```python
from build123d import *

# Parameters (mm, degrees)
SKETCH1_W            = 37
SKETCH1_H            = 57
SKETCH1_W_2          = 22
SKETCH1_H_2          = 42
BOSS_EXTRUDE1_DEPTH  = 5
M4_CLEARANCE_HOLE1_D = 4.5
SKETCH4_W            = 5
SKETCH4_H            = 57
BOSS_EXTRUDE2_DEPTH  = 30


with BuildPart() as part:
    # Sketch1 → Boss-Extrude1 (new body)
    with BuildSketch(Plane(origin=(0, 0, 0), x_dir=(1, 0, 0), z_dir=(0, 1, 0))):
        Rectangle(SKETCH1_W, SKETCH1_H)
        Rectangle(SKETCH1_W_2, SKETCH1_H_2, mode=Mode.SUBTRACT)
    extrude(amount=BOSS_EXTRUDE1_DEPTH)

    # M4 Clearance Hole1 (through all)
    with Locations(Plane(origin=(0, 5, 0), x_dir=(1, 0, 0), z_dir=(0, 1, 0))):
        with Locations((-6.3, 24.2), (6.3, 24.2), (-6.3, -24.2), (6.3, -24.2)):
            Hole(M4_CLEARANCE_HOLE1_D / 2)

    # Sketch4 → Boss-Extrude2 (add)
    with BuildSketch(Plane(origin=(0, 0, 0), x_dir=(1, 0, 0), z_dir=(0, 1, 0))):
        with Locations((-21, 0)):
            Rectangle(SKETCH4_W, SKETCH4_H)
        with Locations((21, 0)):
            Rectangle(SKETCH4_W, SKETCH4_H)
    extrude(amount=BOSS_EXTRUDE2_DEPTH)


solid = part.part
```
Verification items for the finished model (mm, model axes). A direction names the side the tool comes from. Coordinates: 2 decimals unless noted, no trailing zeros. Order: outer loops, then holes, each group sorted by start corner. A loop starts at its lowest first (then second) coordinate and runs counter-clockwise, first axis right, second up. Notation, with made-up numbers: (56.25, -13.75) - (66.25, -13.75) arc R19 cw to (66.25, -2.75) - close; hole circle Ø9 at (-31, -7). An arc over 180 degrees is marked (long way). Return JSON: item names as keys, results as strings.
(1) Section check B-B, the plane y = 23.5. Record the cut outline in (x, z).
Filled sheet:
{"outline": "(-23.5, -28.5) - (-18.5, -28.5) - (-18.5, 28.5) - (-23.5, 28.5) - close; (18.5, -28.5) - (23.5, -28.5) - (23.5, 28.5) - (18.5, 28.5) - close"}
(2) Mould release check, pull along Z, two halves, no side actions. Record for faces 4 (the flat face through (11, 2, 0)), 5 (the flat face through (-11, 2, 0)), 6 (the flat face through (-0.3, 4.8, 28.5)), 7 (the flat face through (-18.5, 17, 0)): pulls with the +Z half, pulls with the -Z half, needs draft (parallel to the pull), parting line crosses it, or undercut.
Filled sheet:
{"face 4": "undercut", "face 5": "undercut", "face 6": "pulls with the +Z half", "face 7": "needs draft"}
(3) Section check C-C, the plane x = -6.3. Record the cut outline in (y, z).
Filled sheet:
{"outline": "(0, -28.5) - (5, -28.5) - (5, -26.45) - (0, -26.45) - close; (0, -21.95) - (5, -21.95) - (5, -21) - (0, -21) - close; (0, 21) - (5, 21) - (5, 21.95) - (0, 21.95) - close; (0, 26.45) - (5, 26.45) - (5, 28.5) - (0, 28.5) - close"}
(4) Access from +Z, -Z, +X, -X, +Y, -Y to the whole of each face (thin tool, end or side, straight path). Record for faces 1 (the flat face through (0, 2, 21)), 2 (the flat face through (-0.3, 4.8, -28.5)), 3 (the flat face through (-13, 5, 0)).
Filled sheet:
{"face 1": "+Y, -Y", "face 2": "-Z, +X, -X, +Y, -Y", "face 3": "+Z, -Z, +Y"}
(5) Section check A-A, the plane z = 8.5. Record the cut outline in (x, y), and give its area (3 significant figures).
Filled sheet:
{"outline": "(-23.5, 0) - (-11, 0) - (-11, 5) - (-18.5, 5) - (-18.5, 30) - (-23.5, 30) - close; (11, 0) - (23.5, 0) - (23.5, 30) - (18.5, 30) - (18.5, 5) - (11, 5) - close", "area": "375 mm^2"}
(6) Section check D-D, the plane z = -24.2. Record the cut outline in (x, y).
Filled sheet:
{"outline": "(-23.5, 0) - (-8.55, 0) - (-8.55, 5) - (-18.5, 5) - (-18.5, 30) - (-23.5, 30) - close; (-4.05, 0) - (4.05, 0) - (4.05, 5) - (-4.05, 5) - close; (8.55, 0) - (23.5, 0) - (23.5, 30) - (18.5, 30) - (18.5, 5) - (8.55, 5) - close"}
(7) Go/stop test with a flat-tipped pin: pin 1 (18.5 mm diameter, centred on x = -6, z = -5.5, fed in from +Y). Record where the tip stops, or that it passes through.
Filled sheet:
{"pin 1": "stops at y = 5"}
(8) Thickness scan on line 1 along Z through (x, y) = (-6.3, 1.5); line 2 along X through (y, z) = (3.75, 24.2); line 3 along X through (y, z) = (13.25, -22). Record the ranges inside material, lowest first.
Filled sheet:
{"line 1": "z = -28.5 to -26.45, -21.95 to -21, 21 to 21.95, 26.45 to 28.5", "line 2": "x = -23.5 to -8.55, -4.05 to 4.05, 8.55 to 23.5", "line 3": "x = -23.5 to -18.5, 18.5 to 23.5"}
